```python
from build123d import *

# Parameters (mm, degrees)
SKETCH1_R           = 2.15
BOSS_EXTRUDE1_DEPTH = 12.7
FILLET1_R           = 6
FILLET2_R           = 6.35
CUT_EXTRUDE1_REACH  = 52.979
SKETCH2_R           = 2.15
CUT_EXTRUDE2_DEPTH  = 4
FILLET3_R           = 1


with BuildPart() as part:
    # Sketch1 → Boss-Extrude1 (new body)
    with BuildSketch(Plane(origin=(0, 0, 0), x_dir=(0, 0, -1), z_dir=(1, 0, 0))):
        Polygon((-38.1, 25.4), (38.1, 25.4), (38.1, 15.4), (12.7, 15.4), (0, -16.003709137), (-12.7, 15.4), (-38.1, 15.4), align=None)
        Circle(SKETCH1_R, mode=Mode.SUBTRACT)
    extrude(amount=BOSS_EXTRUDE1_DEPTH)

    # Fillet1
    fillet1_edges = [part.edges().sort_by_distance(p)[0] for p in [
        (6.35, 15.4, -12.7),
        (6.35, -16.003709137, 0),
        (6.35, 15.4, 12.7),
    ]]
    fillet(fillet1_edges, radius=FILLET1_R)

    # Fillet2
    fillet2_edges = [part.edges().sort_by_distance(p)[0] for p in [
        (0, 20.4, -38.1),
        (12.7, 20.4, -38.1),
        (0, 20.4, 38.1),
        (12.7, 20.4, 38.1),
    ]]
    fillet(fillet2_edges, radius=FILLET2_R - 0.0001)  # a hair under: the kernel refuses the full size

    # Sketch2 → Cut-Extrude1 (cut, up to next)
    with BuildSketch(Plane(origin=(0, 25.4, 0), x_dir=(1, 0, 0), z_dir=(0, 1, 0)), mode=Mode.PRIVATE) as cut_extrude1_sk1:
        with Locations(Location((6.35, -31.75, 0), (0, 0, 270))):
            Circle(SKETCH2_R)
    cut_extrude1_tool1 = extrude(cut_extrude1_sk1.sketch, amount=-CUT_EXTRUDE1_REACH, mode=Mode.PRIVATE) & part.part
    # Sketch2 → Cut-Extrude1 (cut, up to next)
    with BuildSketch(Plane(origin=(0, 25.4, 0), x_dir=(1, 0, 0), z_dir=(0, 1, 0)), mode=Mode.PRIVATE) as cut_extrude1_sk2:
        with Locations(Location((6.35, 31.75, 0), (0, 0, 270))):
            Circle(SKETCH2_R)
    cut_extrude1_tool2 = extrude(cut_extrude1_sk2.sketch, amount=-CUT_EXTRUDE1_REACH, mode=Mode.PRIVATE) & part.part
    add(cut_extrude1_tool1.solids().sort_by_distance((6.35, 25.4, 31.75))[0], mode=Mode.SUBTRACT)
    add(cut_extrude1_tool2.solids().sort_by_distance((6.35, 25.4, -31.75))[0], mode=Mode.SUBTRACT)

    # Sketch3 → Cut-Extrude2 (cut)
    with BuildSketch(Plane.ZY):
        Polygon((0, 4.734272207), (-4.1, 2.367136104), (-4.1, -2.367136104), (0, -4.734272207), (4.1, -2.367136104), (4.1, 2.367136104), align=None)
    extrude(amount=-CUT_EXTRUDE2_DEPTH, mode=Mode.SUBTRACT)

    # Fillet3
    fillet3_edges = [part.edges().sort_by_distance(p)[0] for p in [
        (0, 15.4, -24.247854145),
        (12.7, 15.4, -24.247854145),
        (0, 4.7, -8.372804145),
        (12.7, 4.7, -8.372804145),
        (0, 4.7, 8.372804145),
        (12.7, 4.7, 8.372804145),
        (0, -6, 0),
        (12.7, -6, 0),
        (0, 14.374779952, -13.391273121),
        (12.7, 14.374779952, -13.391273121),
        (0, 14.374779952, 13.391273121),
        (12.7, 14.374779952, 13.391273121),
        (0, 25.4, 0),
        (12.7, 25.4, 0),
        (10.84015735, 25.4, 36.24015735),
        (1.85984265, 25.4, 36.24015735),
        (10.84015735, 25.4, -36.24015735),
        (1.85984265, 25.4, -36.24015735),
        (0, 15.4, 24.247854145),
        (10.84015735, 15.4, -36.24015735),
        (1.85984265, 15.4, -36.24015735),
        (12.7, 15.4, 24.247854145),
        (10.84015735, 15.4, 36.24015735),
        (1.85984265, 15.4, 36.24015735),
    ]]
    fillet(fillet3_edges, radius=FILLET3_R)


solid = part.part
```
Source: CAD feature listing. Evaluate the final solid. Frame: model axes, mm. A direction names the side the tool comes from. Give positions to 0.01 mm unless a question says otherwise; leave off trailing zeros. Loops run counter-clockwise (first coordinate to the right, second up) from the corner with the lowest first, then second, coordinate; pieces in that order, holes last. Notation, with made-up numbers: (36.25, 87) -> (73.25, 87) arc R19 cw to (73.25, 110) -> close; hole circle Ø7 at (81, 83.5). An arc over 180 degrees is marked (long way). Use a Markdown table: item, result. Add a question column.
(1) Section query A-A (z = 24). Output: boundary loops of the cut face in (x, y).
(2) First-contact query: pin 1 Ø1.2 at (x, y) = (1.5, 0.5) entering from +Z; pin 2 Ø5.5 at (x, z) = (9, 23) entering from -Y; pin 3 Ø5 at (x, y) = (1.5, 0) entering from -Z. Flat tips, straight axial feed; report the tip coordinate or a pass-through.
(3) Ray query, line 1 (X direction, y = 18, z = -31.75); line 2 (X direction, y = 23, z = -31); line 3 (Y direction, x = 8.25, z = -20.5). Return the intervals inside material, ascending.
(4) Section query B-B (x = 7.5). Count the separate pieces of the cut face and the enclosed holes in it, then the cut area to 3 significant figures.
(5) Access query for faces 4 (the face through (6.275, 4.797, -8.412)), 5 (the face through (2, 0, 4.1)). Directions: +Z, -Z, +X, -X, +Y, -Y. A direction counts if a zero-diameter tool reaches every point of the face in a straight line with its end or side. Return the directions, or none.
(6) Pull-direction query (Z, two-part tool) for faces 1 (the face through (6, 25.4, 1)), 2 (the face through (6.42, 14.4, 13.43)), 3 (the face through (1.97, 3.57, -2.02)); classes: +Z half, -Z half, draft (parallel to the pull), parting line (faces both ways), or undercut.
Checked values:
| question | item | result |
|---|---|---|
| 1 | outline | (0, 16.4) arc R1 ccw to (1, 15.4) -> (11.7, 15.4) arc R1 ccw to (12.7, 16.4) -> (12.7, 24.4) arc R1 ccw to (11.7, 25.4) -> (1, 25.4) arc R1 ccw to (0, 24.4) -> close |
| 2 | pin 1 | z = 6.92 |
| 2 | pin 2 | y = 15.4 |
| 2 | pin 3 | z = -7.48 |
| 3 | line 1 | 0 to 4.2, 8.5 to 12.7 |
| 3 | line 2 | 0 to 4.34, 8.36 to 12.7 |
| 3 | line 3 | 15.4 to 25.4 |
| 4 | separate pieces | 3 |
| 4 | enclosed holes | 1 |
| 4 | area | 1,030 mm^2 |
| 5 | face 4 | -Z, +X, -X, -Y |
| 5 | face 5 | -X |
| 6 | face 1 | draft |
| 6 | face 2 | +Z half |
| 6 | face 3 | undercut |
